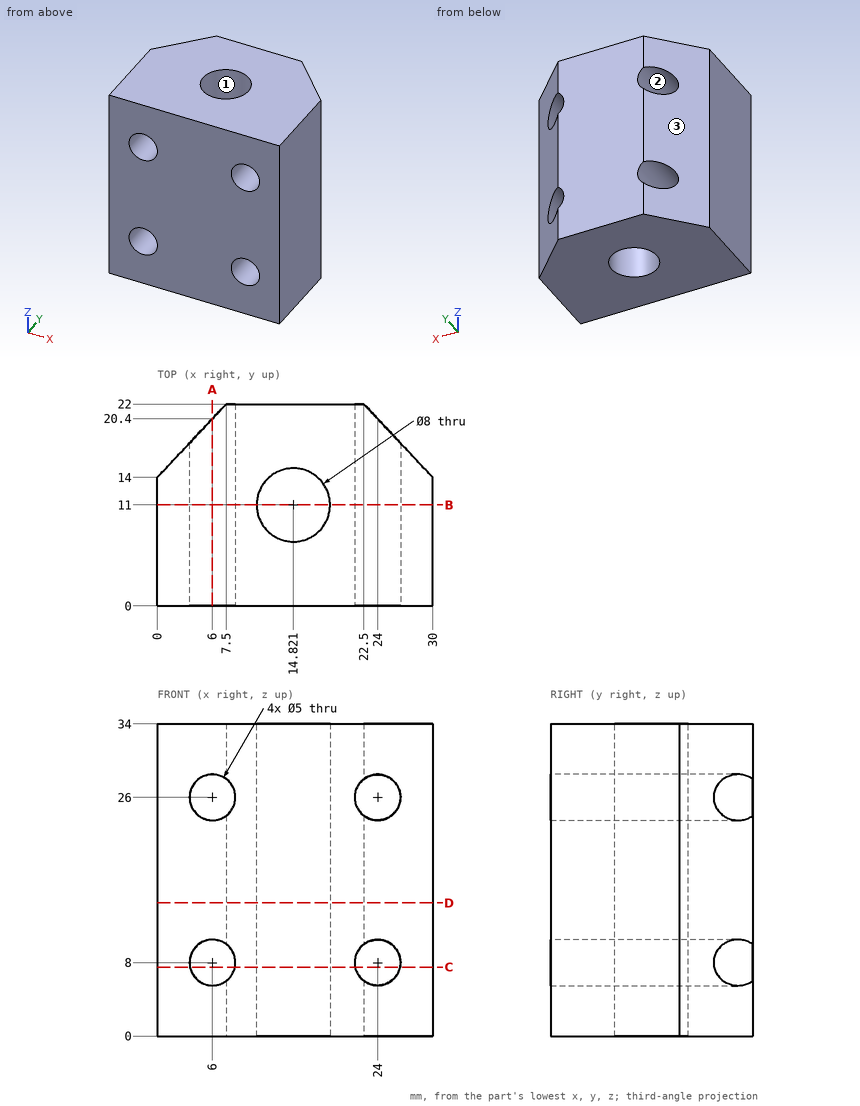
Source: three-view drawing plus pictorial views. Frame: mm from the lowest corner of the part. Give positions to 0.01 mm unless a question says otherwise; leave off trailing zeros. Write each loop counter-clockwise with the first axis right and the second up, starting at its lowest first coordinate (ties: lowest second). Pieces come first, ordered by that corner, then holes.
(1) Cut plane B-B, the plane y = 11. Return loops of the section in (x, z).
(2) Mould query, pull axis Y, two halves, no side actions, for the marked faces 1, 2 and 3. Classes: released by +Y, released by -Y, zero draft, split by the parting line, or undercut.
(3) Cut plane A-A, the plane x = 6. Return loops of the section in (y, z).
(4) Cut plane C-C, the plane z = 7.5. Return loops of the section in (x, y).
(5) First-contact query: P1, Ø1.5, axis at x = 27, z = 27, coming from the +Y side (1 decimal); P2, Ø3, axis at y = 16, z = 29.5, coming from the +X side. Flat tips, straight axial feed; report the tip coordinate or a pass-through.
(6) Ray query, line 1 (Z direction, x = 6, y = 12); line 2 (Y direction, x = 15, z = 14) (1 decimal); line 3 (X direction, y = 12.75, z = 8) (1 decimal). Return the intervals inside material, ascending.
(7) Cut plane D-D, the plane z = 14.5. Return loops of the section in (x, y), then the cut area to 3 significant figures.
Values follow:
1. outline: (0, 0) - (10.82, 0) - (10.82, 34) - (0, 34) - close; (18.82, 0) - (30, 0) - (30, 34) - (18.82, 34) - close; hole circle Ø5 at (6, 8); hole circle Ø5 at (6, 26); hole circle Ø5 at (24, 8); hole circle Ø5 at (24, 26)
2. face 1: undercut
2. face 2: zero draft
2. face 3: released by +Y
3. outline: (0, 0) - (20.4, 0) - (20.4, 5.5) - (0, 5.5) - close; (0, 10.5) - (20.4, 10.5) - (20.4, 23.5) - (0, 23.5) - close; (0, 28.5) - (20.4, 28.5) - (20.4, 34) - (0, 34) - close
4. outline: (0, 0) - (3.55, 0) - (3.55, 17.79) - (0, 14) - close; (8.45, 0) - (21.55, 0) - (21.55, 22) - (8.45, 22) - close; (26.45, 0) - (30, 0) - (30, 14) - (26.45, 17.79) - close; hole circle Ø8 at (14.82, 11)
5. P1: stops at y = 18
5. P2: stops at x = 29.53
6. line 1: z = 0 to 5.5, 10.5 to 23.5, 28.5 to 34
6. line 2: y = 0 to 7, 15 to 22
6. line 3: x = 0 to 3.5, 8.5 to 11.2, 18.4 to 21.5, 26.5 to 30
7. outline: (0, 0) - (30, 0) - (30, 14) - (22.5, 22) - (7.5, 22) - (0, 14) - close; hole circle Ø8 at (14.82, 11)
7. area: 550 mm2
